from build123d import *

# Parameters (mm, degrees)
F0_R     = 11.05
F1_DEPTH = 7


with BuildPart() as f1:
    # F0 (on Top) → F1 (new body)
    with BuildSketch(Plane.XY):
        with BuildLine():
            ThreePointArc((-12.6831392694, 4.7686977545), (-2.4234234979, -13.3315234895), (13.55, 0))
            ThreePointArc((13.55, 0), (13.1027192195, 3.4527161853), (11.7904060434, 6.6774864532))
            add(Edge.make_bspline(
                [(11.5297847403, 7.1180449452), (11.6132861066, 6.969341391), (11.7001892822, 6.8225044208), (11.7904060434, 6.6774864532)],
                knots=[0.4974758981, 0.4974758981, 0.4974758981, 0.4974758981, 0.5104096373, 0.5104096373, 0.5104096373, 0.5104096373], degree=3))
            ThreePointArc((11.5297847403, 7.1180449452), (1.1469220688, 13.5013728846), (-10.1639023184, 8.9608922359))
            add(Edge.make_bspline(
                [(-10.1639023184, 8.9608922359), (-10.7500939319, 7.4698745289), (-11.6129235501, 6.081120856), (-12.6831392694, 4.7686977545)],
                knots=[0.4943184599, 0.4943184599, 0.4943184599, 0.4943184599, 0.6210165425, 0.6210165425, 0.6210165425, 0.6210165425], degree=3))
        make_face()
        Circle(F0_R, mode=Mode.SUBTRACT)
        with BuildLine():
            ThreePointArc((11.7904060434, 6.6774864532), (13.1027192195, 3.4527161853), (13.55, 0))
            ThreePointArc((13.55, 0), (-2.4234234979, -13.3315234895), (-12.6831392694, 4.7686977545))
            add(Edge.make_bspline(
                [(-12.6831392694, 4.7686977545), (-15.884403608, 0.8429347549), (-20.9412495964, -2.399862478), (-26.0002209429, -5.6537765206)],
                knots=[0.6210165425, 0.6210165425, 0.6210165425, 0.6210165425, 1, 1, 1, 1], degree=3))
            ThreePointArc((-26.0002209429, -5.6537765206), (-20.0363711479, -10.649419061), (-17.8030151047, -18.1016717106))
            ThreePointArc((-17.8030151047, -18.1016717106), (-18.1329053392, -21.0734048392), (-19.1065129332, -23.9004374898))
            add(Edge.make_bspline(
                [(-19.1065129332, -23.9004374898), (-12.7337335325, -19.9495363252), (-0.2067317894, -12.1959048864), (12.344888234, -18.8150479155), (18.4126389706, -22.1202741428)],
                knots=[0, 0, 0, 0, 0.5079978735, 1, 1, 1, 1], degree=3))
            ThreePointArc((18.4126389706, -22.1202741428), (20.4851117611, -10.0090097929), (31.4943521465, -4.5524088583))
            add(Edge.make_bspline(
                [(11.7904060434, 6.6774864532), (15.2054475833, 1.1880144624), (23.3685436118, -1.6949988805), (31.4943521465, -4.5524088583)],
                knots=[0.5104096373, 0.5104096373, 0.5104096373, 0.5104096373, 1, 1, 1, 1], degree=3))
        make_face()
        with BuildLine():
            ThreePointArc((-10.1639023184, 8.9608922359), (1.1469220688, 13.5013728846), (11.5297847403, 7.1180449452))
            add(Edge.make_bspline(
                [(11.9294824461, 29.7776178927), (10.1390437597, 21.3188304105), (8.3180362773, 12.8376928177), (11.5297847403, 7.1180449452)],
                knots=[0, 0, 0, 0, 0.4974758981, 0.4974758981, 0.4974758981, 0.4974758981], degree=3))
            ThreePointArc((11.9294824461, 29.7776178927), (0.164433974, 22.6543411898), (-11.7700234604, 29.4899949467))
            add(Edge.make_bspline(
                [(-11.7700234604, 29.4899949467), (-9.8007963488, 22.152111828), (-7.8768484836, 14.7781671429), (-10.1639023184, 8.9608922359)],
                knots=[0, 0, 0, 0, 0.4943184599, 0.4943184599, 0.4943184599, 0.4943184599], degree=3))
        make_face()
        with BuildLine():
            ThreePointArc((44.9030151047, -18.1016717106), (40.9841525484, -8.5704760069), (31.4943521465, -4.5524088583))
            ThreePointArc((31.4943521465, -4.5524088583), (20.4851117611, -10.0090097929), (18.4126389706, -22.1202741428))
            ThreePointArc((18.4126389706, -22.1202741428), (33.3853048703, -31.4983988597), (44.9030151047, -18.1016717106))
        make_face()
        with Locations((31.3530151047, -18.1016717106)):
            Circle(F0_R, mode=Mode.SUBTRACT)
        with BuildLine():
            ThreePointArc((-17.8030151047, -18.1016717106), (-20.0363711479, -10.649419061), (-26.0002209429, -5.6537765206))
            ThreePointArc((-26.0002209429, -5.6537765206), (-44.028541405, -22.8905685576), (-19.1065129332, -23.9004374898))
            ThreePointArc((-19.1065129332, -23.9004374898), (-18.1329053392, -21.0734048392), (-17.8030151047, -18.1016717106))
        make_face()
        with Locations((-31.3530151047, -18.1016717106)):
            Circle(F0_R, mode=Mode.SUBTRACT)
        with BuildLine():
            ThreePointArc((-11.7700234604, 29.4899949467), (0.164433974, 22.6543411898), (11.9294824461, 29.7776178927))
            ThreePointArc((11.9294824461, 29.7776178927), (13.1386260154, 32.8898850425), (13.55, 36.2033434212))
            ThreePointArc((13.55, 36.2033434212), (-3.472656196, 49.3007919874), (-11.7700234604, 29.4899949467))
        make_face()
        with Locations((0, 36.2033434212)):
            Circle(F0_R, mode=Mode.SUBTRACT)
    extrude(amount=F1_DEPTH)


solid = f1.part
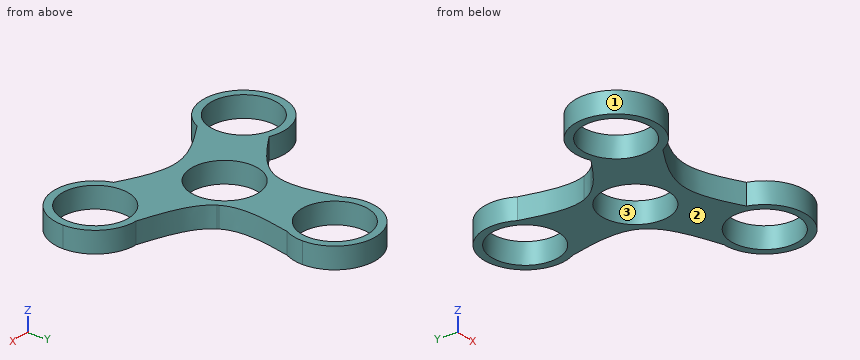
Model file for the job. Use its own axes, mm. Face numbers are marked on the shaded views. Give positions to 0.01 mm unless a question says otherwise; leave off trailing zeros. Order: outer loops, then holes, each group sorted by start corner. A loop starts at its lowest first (then second) coordinate and runs counter-clockwise, first axis right, second up. Notation, with made-up numbers: (-16.5, -5.75) - (25.5, -5.75) arc R12 cw to (25.5, 12.25) - close; hole circle Ø10 at (-17.75, -24.75). An arc over 180 degrees is marked (long way). Write item = value, one per line. Start each with the question number.
1. Cut at D-D, the plane x = 0. State how many separate pieces and enclosed holes the cut face has, and give its area (3 significant figures).
2. Cut at C-C, the plane y = 39. List the corners of the cut face in (x, z).
3. Cut at A-A, the plane x = -36. List the corners of the cut face in (y, z), and give its area (3 significant figures).
4. Cut at B-B, the plane y = -12.5. List the corners of the cut face in (x, z), and give its area (3 significant figures).
5. Drop flat-ended pins along their axis: P1, Ø13.5, axis at x = 0, y = 36.2, coming from the +Z side; P2, Ø4, axis at y = -10, z = 3.5, coming from the +X side; P3, Ø4, axis at x = -6, z = 4, coming from the -Y side; P4, Ø1.5, axis at y = 22.5, z = 1, coming from the -X side. Give the stop position or say it passes through.
6. Probe line 1 along Y through (x, z) = (-8, 2); line 2 along Y through (x, z) = (-5, 2.75); line 3 along X through (y, z) = (-20, 1.5). List the from-to ranges inside material, lowest first.
7. Two-plate mould, pull along Y, no slides. Class the marked faces 1, 2 and 3: pulls with the +Y half, pulls with the -Y half, needs draft (parallel to the pull), parting line crosses it, or undercut.
Taken from the geometry:
q1.separate_pieces = 3
q1.enclosed_holes = 0
q1.area = 149 mm²
q2.outline = (-13.26, 0) - (-10.69, 0) - (-10.69, 7) - (-13.26, 7) - close; (10.69, 0) - (13.26, 0) - (13.26, 7) - (10.69, 7) - close
q3.outline = (-30.83, 0) - (-28.13, 0) - (-28.13, 7) - (-30.83, 7) - close; (-8.08, 0) - (-5.37, 0) - (-5.37, 7) - (-8.08, 7) - close
q3.area = 37.8 mm²
q4.outline = (-43.69, 0) - (-40.88, 0) - (-40.88, 7) - (-43.69, 7) - close; (-21.83, 0) - (21.83, 0) - (21.83, 7) - (-21.83, 7) - close; (40.88, 0) - (43.69, 0) - (43.69, 7) - (40.88, 7) - close
q4.area = 345 mm²
q5.P1 = through
q5.P2 = 43.45
q5.P3 = -17.75
q5.P4 = -10.2
q6.line_1 = -17.75 to -7.62, 7.62 to 28.58, 43.83 to 47.14
q6.line_2 = -16.66 to -9.85, 9.85 to 26.35, 46.06 to 48.8
q6.line_3 = -44.77 to -42.24, -20.47 to -12.57, 14.43 to 20.47, 42.24 to 44.77
q7.face_1 = parting line crosses it
q7.face_2 = needs draft
q7.face_3 = undercut
